Autodesk Fusion 360 part; units mm, degrees
sketch "Sketch1" plane through (0, 0, 0) normal (0, 1, 0) x (1, 0, 0)
  line L0 (10, 0) -> (50, 0)
  line L1 (-50, 0) -> (-50, 20)
  line L2 (-50, 20) -> (-38, 20)
  line L3 (-38, 20) -> (-38, 12)
  line L4 (-38, 12) -> (38, 12)
  line L5 (38, 12) -> (38, 20)
  line L6 (38, 20) -> (50, 20)
  line L7 (50, 20) -> (50, 0)
  line L8 (50, 20) -> (50, 0)
  line L9 (50, 0) -> (10, 0)
  line L10 (50, 0) -> (10, 0)
  line L11 (-10, 0) -> (-50, 0)
  line L12 (-10, 0) -> (-10, -24)
  line L13 (-10, -24) -> (10, -24)
  line L14 (10, -24) -> (10, 0)
  dimension "d1" = 50
  dimension "d2" = 100
  dimension "d3" = 20
  dimension "d4" = 12
  dimension "d5" = 8
  dimension "d6" = 76
  dimension "d7" = 8
  dimension "d8" = 20
  dimension "d9" = 40
  dimension "d13" = 24
  dimension "d14" = 20
extrude "Extrude1" add sketch "Sketch1" along normal blind 40
sketch "Sketch2" plane through (0, 0, 0) normal (0, 0, 1) x (-1, 0, 0)
  line L0 (-10, 0) -> (-50, 0)
  line L1 (-50, 0) -> (-50, -40)
  line L2 (-50, -40) -> (-10, -40)
  line L3 (-10, -40) -> (-10, 0)
  line L4 (-30, -40) -> (-30, 0)
  circle A0 centre (-30, -20) radius 6
  line L5 (50, 0) -> (30, 0)
  line L6 (30, 0) -> (30, -40)
  circle A1 centre (30, -20) radius 6
  dimension "d17" = 12
  dimension "d18" = 20
  dimension "d19" = 12
extrude "Extrude2" cut sketch "Sketch2" against normal blind 20 contours L4 A0 | L4 A0
sketch "Sketch3" plane through (0, 0, 0) normal (0, 0, 1) x (-1, 0, 0)
  line L0 (50, 0) -> (10, 0)
  line L1 (10, 0) -> (10, -40)
  line L2 (10, -40) -> (50, -40)
  line L3 (50, -40) -> (50, 0)
  line L4 (50, 0) -> (30, 0)
  line L5 (30, 0) -> (30, -40)
  circle A0 centre (30, -20) radius 6
  dimension "d22" = 12
extrude "Extrude3" cut sketch "Sketch3" against normal blind 20 contours L5 A0 | L5 A0
sketch "Sketch4" plane through (10, 0, 0) normal (1, 0, 0) x (0, 1, 0)
  line L0 (0, 24) -> (0, 0)
  line L1 (0, 0) -> (40, 0)
  line L2 (40, 0) -> (40, 24)
  line L3 (40, 24) -> (0, 24)
  circle A0 centre (20, 24) radius 20
  dimension "d25" = 40
extrude "Extrude4" add sketch "Sketch4" against normal blind 20 contours L3 A0 picked at (20.4982, 30.648)
sketch "Sketch5" plane through (10, 0, 0) normal (1, 0, 0) x (0, 1, 0)
  line L0 (0, 24) -> (0, 0)
  line L1 (0, 0) -> (40, 0)
  line L2 (40, 0) -> (40, 24)
  arc A0 (40, 24) -> (0, 24) centre (20, 24) ccw
  line L3 (0, 0) -> (0, 25)
  line L4 (0, 25) -> (40, 25)
  circle A1 centre (20, 25) radius 12
  dimension "d28" = 40
  dimension "d29" = 24
extrude "Extrude5" cut sketch "Sketch5" against normal blind 20 contours L4 A1 | L4 A1
sketch "Sketch6" plane through (0, 0, 0) normal (0, -1, 0) x (1, 0, 0)
  line L0 (-10, 24) -> (-10, 0)
  line L1 (-10, 0) -> (-50, 0)
  line L2 (-50, 0) -> (-50, -20)
  line L3 (-50, -20) -> (-38, -20)
  line L4 (-38, -20) -> (-38, -12)
  line L5 (-38, -12) -> (38, -12)
  line L6 (38, -12) -> (38, -20)
  line L7 (38, -20) -> (50, -20)
  line L8 (50, -20) -> (50, 0)
  line L9 (50, 0) -> (10, 0)
  line L10 (10, 0) -> (10, 24)
  line L11 (10, 24) -> (-10, 24)
Can you work these out from the model? Positions are in its coordinate system, mm. A direction names the side the tool comes from. Round coordinates to 2 decimals unless told otherwise and drop trailing zeros. Loops run counter-clockwise (first coordinate to the right, second up) from the corner with the lowest first, then second, coordinate; pieces in that order, holes last. Notation, with made-up numbers: M 51.25,39 L 83.25,39 A27 ccw 83.25,74 Z; hole C 3,47.25 d8. An arc over 180 degrees is marked long. Answer as a JSON object with one key per item and string values. Group by question number.
Q1. Imagine slicing it at A-A, the plane x = 30. Please give me the cut outline in (y, z).
Q2. Imagine slicing it at C-C, the plane z = 22.5. Please give me the cut outline in (x, y), then the cut area to 3 significant figures.
Q3. Imagine slicing it at D-D, the plane x = -8.5. Please give me the cut outline in (y, z).
Q4. We'd pull the mould along Z, two halves only. Please class faces 1 (the flat face through (-44, 20, -20)), 2 (the cylindrical face through (0, 20, 44)), 3 (the flat face through (0, 0, -1)), 4 (the cylindrical face through (0.14, 17.399, 13.285)): +Z half, -Z half, draft (parallel to the pull), parting line (faces both ways), or undercut.
Q5. Will these pins go through, and if not, where does the flat tip stop? pin 1 (3 mm diameter, centred on x = -25, y = 31.5, fed in from -Z); pin 2 (20 mm diameter, centred on x = 23, y = 29, fed in from +Z); pin 3 (8 mm diameter, centred on y = 6.5, z = 28.5, fed in from +X).
Q6. Imagine slicing it at B-B, the plane y = 20. Please give me the cut outline in (x, z).
Q7. Please list where these lines run through material, in increasing order: L1, parallel to Y at x = 30, z = -2.5; L2, parallel to X at y = 20, z = -3.25; L3, parallel to X at y = 3, z = -17.
Q8. On a 3-axis mill with a long thin cutter (end or side, diameter ignored), from which of +Z, -Z, +X, -X, +Y, -Y can I reach the whole of each face in a straight line? I mean faces 5 (the flat face through (38, 20, -16)), 6 (the flat face through (25, 15, 0)), 7 (the flat face through (-25, 15, 0)). Say none if no direction works.
Findings:
{
 "1": {"outline": "M 0,-12 L 14,-12 L 14,0 L 0,0 Z; M 26,-12 L 40,-12 L 40,0 L 26,0 Z"},
 "2": {"outline": "M -10,0 L 10,0 L 10,8.26 L -10,8.26 Z; M -10,31.74 L 10,31.74 L 10,40 L -10,40 Z", "area": "331 mm2"},
 "3": {"outline": "M 0,-12 L 40,-12 L 40,24 A20 ccw 0,24 Z; hole C 20,25 d24"},
 "4": {"face 1": "-Z half", "face 2": "+Z half", "face 3": "draft", "face 4": "undercut"},
 "5": {"pin 1": "stops at z = -12", "pin 2": "stops at z = 0", "pin 3": "stops at x = 10"},
 "6": {"outline": "M -50,-20 L -38,-20 L -38,-12 L -36,-12 L -36,0 L -50,0 Z; M -24,-12 L 24,-12 L 24,0 L 10,0 L 10,13 L -10,13 L -10,0 L -24,0 Z; M -10,37 L 10,37 L 10,44 L -10,44 Z; M 36,-12 L 38,-12 L 38,-20 L 50,-20 L 50,0 L 36,0 Z"},
 "7": {"L1": "y = 0 to 14, 26 to 40", "L2": "x = -50 to -36, -24 to 24, 36 to 50", "L3": "x = -50 to -38, 38 to 50"},
 "8": {"face 5": "-Z, +Y, -Y", "face 6": "+Z, +X, +Y, -Y", "face 7": "+Z, -X, +Y, -Y"}
}
